Read the model definition and answer for the solid it produces. Units are mm, in the model's axes. A direction names the side the tool comes from. Coordinates: 2 decimals unless noted, no trailing zeros. Loops run counter-clockwise (first coordinate to the right, second up) from the corner with the lowest first, then second, coordinate; pieces in that order, holes last. Notation, with made-up numbers: (-21, 44.25) -> (13, 44.25) arc R12 ccw to (13, 62.25) -> close; hole circle Ø2 at (-39.75, 80.25). An arc over 180 degrees is marked (long way). Answer as a JSON object with one key per item and string values. Group by question number.
Q1. For faces 1 (the cylindrical face through (-9.318, -601.066, 70.173)), 2 (the flat face through (-1, -601, 0)), 3 (the flat face through (51.679, -601.066, 17.086)), determine the directions among +Z, -Z, +X, -X, +Y, -Y from which every point of the face is accessible in a straight line to the end or side of a thin tool.
Q2. The part is cut by section C-C on x = -53. Write down the section's boundary in (y, z), and give its area (3 significant figures).
Q3. Each of these flat-tipped pins is pushed along its axis until it touches: P1, Ø8, axis at y = -427, z = 111, coming from the -X side; P2, Ø8, axis at x = -30.5, y = -509, coming from the -Z side; P3, Ø12, axis at y = -794, z = 137, coming from the +X side. Where does it stop, or does it pass through?
Q4. The part is cut by section B-B on z = 82. Write down the section's boundary in (x, y).
Q5. Straight lines are drawn through the part: line 1 along X through (y, z) = (-1070.5, 119); line 2 along X through (y, z) = (-411, 91.5); line 3 along Z through (x, y) = (35, -365.5). For each, find the intervals that lie inside material, in ascending order. Write a range as [from, to].
Q6. Determine the mould class of faces 4 (the cylindrical face through (9.374, -601.066, 69.372)), 5 (the flat face through (0, -601, 180.975)), 6 (the flat face through (-6, -1219.2, 84)) for opening direction Z: released by +Z, released by -Z, zero draft, split by the parting line, or undercut.
from build123d import *

# Parameters (mm, degrees)
F1_DEPTH = 1219.2
F2_R     = 3.175
F3_R     = 22.225
F4_R     = 19.05


with BuildPart() as f1:
    # F0 (on Front) → F1 (new body)
    with BuildSketch(Plane.XZ):
        Polygon((-76.2, 10.880936), (-76.2, 0), (76.2, 0), (76.2, 10.880936), (14.762829, 26.42693), (8.334375, 28.053579), (-8.334375, 28.053579), (-14.762829, 26.42693), align=None)
        with BuildLine():
            ThreePointArc((-8.334375, 98.425), (-9.944679, 62.282756), (-14.762829, 26.42693))
            Line((-14.762829, 26.42693), (-8.334375, 28.053579))
            Line((-8.334375, 28.053579), (-8.334375, 98.425))
        make_face()
        with BuildLine():
            Line((8.334375, 28.053579), (14.762829, 26.42693))
            ThreePointArc((14.762829, 26.42693), (9.944679, 62.282756), (8.334375, 98.425))
            Line((8.334375, 98.425), (8.334375, 28.053579))
        make_face()
        Polygon((-8.334375, 98.425), (-8.334375, 28.053579), (0, 30.1625), (8.334375, 28.053579), (8.334375, 98.425), (8.334375, 131.490171), (0, 129.38125), (-8.334375, 131.490171), align=None)
        Polygon((-11.161954, 132.205659), (-8.334375, 131.490171), (8.334375, 131.490171), (11.161954, 132.205659), (38.1, 139.022032), (-38.1, 139.022032), align=None)
        with BuildLine():
            Line((-37.607689, 161.405181), (-38.1, 139.022032))
            Line((-38.1, 139.022032), (38.1, 139.022032))
            Line((38.1, 139.022032), (37.607689, 161.405181))
            ThreePointArc((37.607689, 161.405181), (32.106429, 174.772303), (19.05, 180.975))
            Line((19.05, 180.975), (-19.05, 180.975))
            ThreePointArc((-19.05, 180.975), (-32.106429, 174.772303), (-37.607689, 161.405181))
        make_face()
        Polygon((8.334375, 131.490171), (-8.334375, 131.490171), (0, 129.38125), align=None)
        with BuildLine():
            Line((8.334375, 131.490171), (8.334375, 98.425))
            ThreePointArc((8.334375, 98.425), (9.042504, 115.374396), (11.161954, 132.205659))
            Line((11.161954, 132.205659), (8.334375, 131.490171))
        make_face()
        with BuildLine():
            ThreePointArc((-11.161954, 132.205659), (-9.042504, 115.374396), (-8.334375, 98.425))
            Line((-8.334375, 98.425), (-8.334375, 131.490171))
            Line((-8.334375, 131.490171), (-11.161954, 132.205659))
        make_face()
        Polygon((0, 30.1625), (-8.334375, 28.053579), (8.334375, 28.053579), align=None)
    extrude(amount=F1_DEPTH)

    # F2
    f2_edges = [f1.edges().sort_by_distance(p)[0] for p in [
        (76.2, -609.6, 10.880936),
        (-76.2, -609.6, 10.880936),
    ]]
    fillet(f2_edges, radius=F2_R)

    # F3
    f3_edges = [f1.edges().sort_by_distance(p)[0] for p in [
        (14.762829, -609.6, 26.42693),
        (-14.762829, -609.6, 26.42693),
    ]]
    fillet(f3_edges, radius=F3_R)

    # F4
    f4_edges = [f1.edges().sort_by_distance(p)[0] for p in [
        (-11.161954, -609.6, 132.205659),
        (11.161954, -609.6, 132.205659),
    ]]
    fillet(f4_edges, radius=F4_R)


solid = f1.part
Final values:
{
 "1": {"face 1": "-X, +Y, -Y", "face 2": "-Z, +X, -X, +Y, -Y", "face 3": "+X, +Y, -Y"},
 "2": {"outline": "(-1219.2, 0) -> (0, 0) -> (0, 16.75) -> (-1219.2, 16.75) -> close", "area": "20,400 mm2"},
 "3": {"P1": "stops at x = -9.01", "P2": "stops at z = 0", "P3": "stops at x = 38.1"},
 "4": {"outline": "(-8.67, -1219.2) -> (8.67, -1219.2) -> (8.67, 0) -> (-8.67, 0) -> close"},
 "5": {"line 1": "x = [-9.38, 9.38]", "line 2": "x = [-8.39, 8.39]", "line 3": "z = [0, 21.31], [138.24, 170.86]"},
 "6": {"face 4": "undercut", "face 5": "released by +Z", "face 6": "zero draft"}
}
